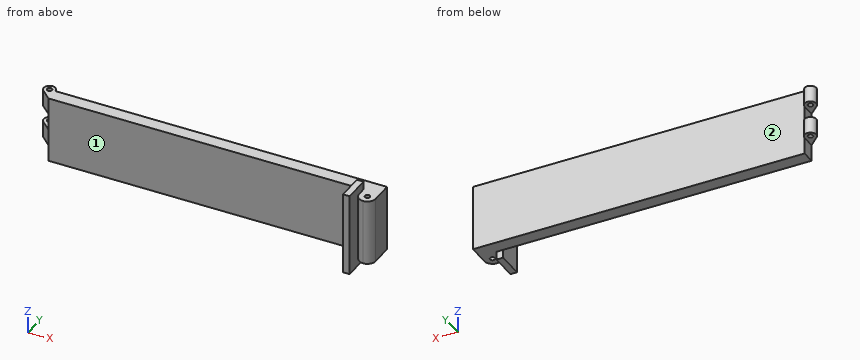
Autodesk Inventor part; units mm, degrees
ref_plane "Arbeitsebene3" through (0, -4, 15) normal (0, -1, 0) x (1, 0, 0)
ref_plane "YZ Plane" through (0, 0, 0) normal (1, 0, 0) x (0, 1, 0)
ref_plane "XZ Plane" through (0, 0, 0) normal (0, 1, 0) x (-1, 0, 0)
sketch "Skizze1" plane through (0, 0, 0) normal (0, 0, 1) x (1, 0, 0)
  line L0 (0, 0) -> (100, 0)
  line L1 (100, 0) -> (100, 4)
  line L2 (100, 4) -> (0, 4)
  line L3 (0, 4) -> (0, 0)
  dimension "d0" = 100
  dimension "d1" = 4
extrude "Extrusion1" add sketch "Skizze1" along normal blind 20
sketch "Skizze2" plane through (0, 0, 0) normal (0, 0, -1) x (-1, 0, 0)
  line L0 (0, 4) -> (0, 0)
  line L1 (-100, 4) -> (0, 4)
  line L2 (0, 4) -> (2.5, 4) construction
  line L3 (1.7678, 5.7678) -> (1.7678, 5.75)
  arc A0 (2.8969, 2.663) -> (0.0178, 4) centre (1.7678, 4) ccw
  line L4 (0, 0) -> (3.0052, 2.7626)
  line L5 (0, 4) -> (0.0179, 4.0179)
  line L6 (1.7499, 5.7499) -> (1.7678, 5.7678)
  circle A1 centre (1.7678, 4) radius 0.75
  dimension "d4" = 2.5
  dimension "d6" = 3.5
  dimension "d9" = 1.5
extrude "Extrusion2" add sketch "Skizze2" against normal blind 20 contours L5 A0 L4 L0 | A1
sketch "Skizze3" plane through (0, 0, 0) normal (0, 0, -1) x (-1, 0, 0)
  point P0 (0, 0)
extrude "Extrusion3" cut sketch "Skizze2" against normal blind 20 contours A1
sketch "Skizze6" plane through (0, 0, 0) normal (0, -1, 0) x (1, 0, 0)
  line L0 (0, 0) -> (0, 20)
  line L1 (0, 20) -> (0, 15)
  line L2 (0, 15) -> (0, 10)
  line L3 (0, 10) -> (0, 5)
  line L4 (0, 5) -> (0, 0)
  line L5 (-3.5178, 0) -> (-0.0179, 0)
  line L6 (0, 0) -> (-3.5178, 0)
  line L7 (-3.5178, 0) -> (-3.5178, 5)
  line L8 (-3.5178, 0) -> (-3.5178, 20)
  line L9 (0, 5) -> (-3.5178, 5)
  line L10 (0, 15) -> (-3.5178, 15)
  line L11 (-3.5178, 15) -> (-3.5178, 10)
  line L12 (0, 10) -> (-3.5178, 10)
  point P0 (-3.0052, 0)
  dimension "d22" = 5
  dimension "d23" = 5
  dimension "d24" = 5
extrude "Extrusion5" cut sketch "Skizze6" against normal blind 50 contours L6 L5 L7 L9 L0 | L12 L8 L10 L0
sketch "Skizze7" plane through (100, 4, 20) normal (1, 0, 0) x (0, 0, -1)
  point P0 (20, -4)
sketch "Skizze10" plane through (0, 0, 20) normal (0, 0, 1) x (1, 0, 0)
  point P0 (0, 0)
sketch "Skizze11" plane through (0, 0, 20) normal (0, 0, 1) x (1, 0, 0)
  line L0 (0, 0) -> (100, 0)
  line L1 (100, 0) -> (95, 0)
  line L2 (95, 0) -> (95, -5)
  line L3 (95, -5) -> (100, -5)
  line L4 (100, -5) -> (100, 0)
  dimension "d28" = 5
  dimension "d29" = 5
extrude "Extrusion6" add sketch "Skizze11" against normal blind 20
sketch "Skizze12" plane through (0, 0, 20) normal (0, 0, 1) x (1, 0, 0)
  line L0 (100, 4) -> (100, -5)
  line L1 (100, -5) -> (97.5, -5)
  line L2 (100, -5) -> (95, -5)
  line L3 (97.5, -5) -> (97.5, -2.5)
  circle A0 centre (97.5, -2.5) radius 0.75
  point P0 (0, 0)
  dimension "d32" = 2.5
  dimension "d33" = 1.5
extrude "Extrusion7" cut sketch "Skizze12" against normal blind 20
fillet "Rundung1" radius 2.5 2 edges at (95, -5, 10) (100, -5, 10)
ref_plane "Arbeitsebene3" through (0, -4, 15) normal (0, -1, 0) x (1, 0, 0)
sketch "Skizze14" plane through (0, -4, 15) normal (0, -1, 0) x (1, 0, 0)
  line L0 (95, 5) -> (95, -15)
  line L1 (0, -15) -> (95, -15)
  line L2 (95, 5) -> (93, 5)
  line L3 (93, 5) -> (93, -15)
  line L4 (93, -15) -> (95, -15)
  line L5 (95, -15) -> (95, 5)
  line L6 (93, 5) -> (95, 5)
  line L7 (95, 5) -> (95, 7.5)
  line L8 (95, 7.5) -> (93, 7.5)
  line L9 (93, 7.5) -> (93, 5)
  line L10 (93, -15) -> (95, -15)
  line L11 (95, -15) -> (95, -17.5)
  line L12 (95, -17.5) -> (93, -17.5)
  line L13 (93, -17.5) -> (93, -15)
  dimension "d39" = 2
  dimension "d40" = 2
  dimension "d41" = 2.5
  dimension "d42" = 2.5
extrude "Extrusion9" add sketch "Skizze14" along normal mid plane 8
properties part number "Hebel_Klemme_unten"
Can you work these out from the model? Positions are in its coordinate system, mm. Face numbers are marked on the shaded views. A direction names the side the tool comes from. Coordinates: 2 decimals unless noted, no trailing zeros. Write each loop counter-clockwise with the first axis right and the second up, starting at its lowest first coordinate (ties: lowest second). Pieces come first, ordered by that corner, then holes.
Q1. Imagine slicing it at C-C, the plane y = -6.25. List the corners of the cut face in (x, z) for me, plus the area to 3 significant figures.
Results found:
outline: (93, -2.5) - (95, -2.5) - (95, 22.5) - (93, 22.5) - close
area: 50.0 mm2
Q2. For P1, Ø8, axis at x = 18, y = 4, coming from the +Z side; P2, Ø4, axis at y = 0, z = 4, coming from the -X side; P3, Ø5, axis at y = -5.5, z = 4, coming from the -X side, each with a flat end and sliding along its axis, tell me the tip position at first contact or that it passes through.
Results found:
P1: stops at z = 20
P2: stops at x = -1.88
P3: stops at x = 93
Q3. Which directions (+Z, -Z, +X, -X, +Y, -Y) give clear straight access to the entire face, cutting with the end or side of a thin tool? Please do the marked faces 1 and 2.
Results found:
face 1: +Z, -Z, -X, -Y
face 2: +Z, -Z, +X, +Y
Q4. Imagine slicing it at B-B, the plane z = 19. Count the separate pieces of the cut face and the enclosed holes in it, plus the area to 3 significant figures.
Results found:
separate pieces: 1
enclosed holes: 2
area: 448 mm2
Q5. Please list where these lines run through material, in increasing order: L1, parallel to Y at x = 97.5, z = 5; L2, parallel to X at y = -1.5, z = 7; L3, parallel to Z at x = 49, y = 0.5.
Results found:
L1: y = -5 to -3.25, -1.75 to 4
L2: x = 93 to 100
L3: z = 0 to 20
Q6. Imagine slicing it at D-D, the plane x = 40. List the corners of the cut face in (y, z) for me, plus the area to 3 significant figures.
Results found:
outline: (0, 0) - (4, 0) - (4, 20) - (0, 20) - close
area: 80.0 mm2
